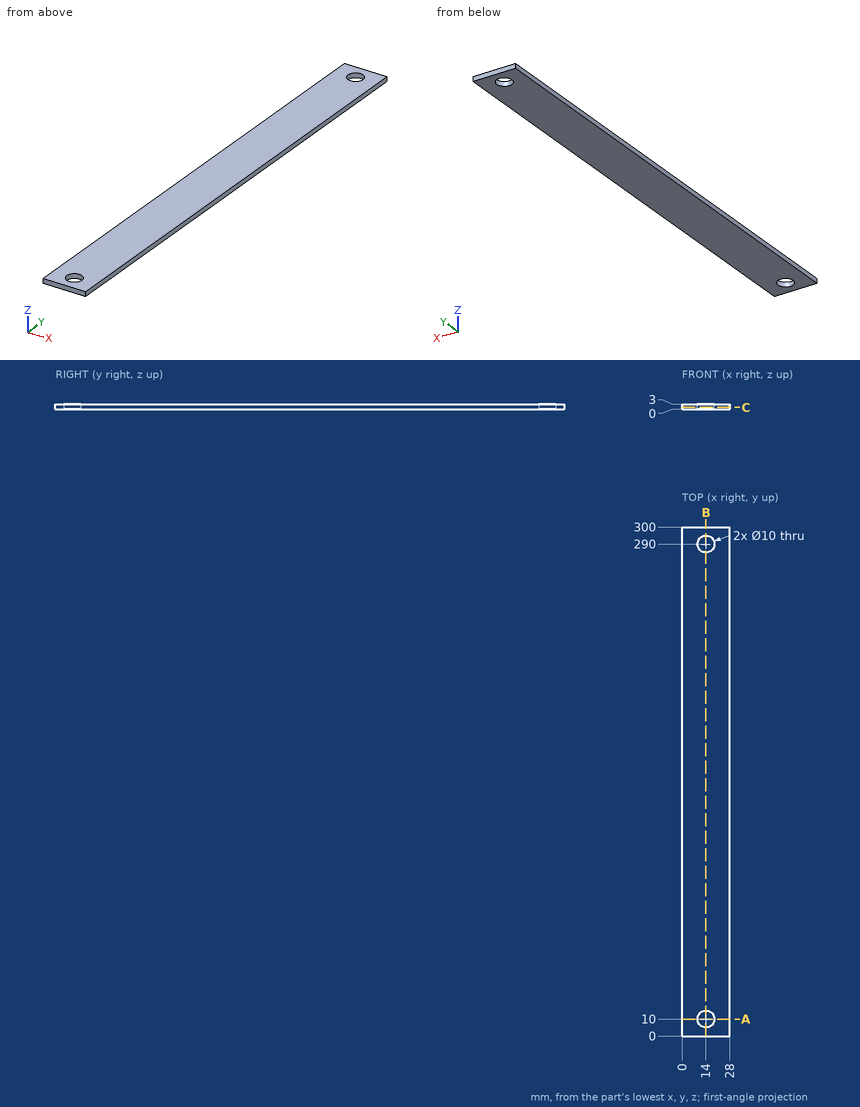
The figure shows three views and two pictorial views of one solid part (mm, origin at its lowest corner). Answer the questions. Give positions to 0.01 mm unless a question says otherwise; leave off trailing zeros. Write each loop counter-clockwise with the first axis right and the second up, starting at its lowest first coordinate (ties: lowest second). Pieces come first, ordered by that corner, then holes. Notation, with made-up numbers: (16.25, 55) -> (43.25, 55) arc R27 ccw to (43.25, 91) -> close; hole circle Ø2 at (41, -25.75). An arc over 180 degrees is marked (long way). Use one line per item in the form item = value.
1) Straight lines are drawn through the part: probe 1 along Y at (x, z) = (14, 1.95); probe 2 along X at (y, z) = (10, 0.95); probe 3 along Y at (x, z) = (13, 2.6). For each, find the intervals that lie inside material, in ascending order.
Result:
probe_1 = 0 to 5, 15 to 285, 295 to 300
probe_2 = 0 to 9, 19 to 28
probe_3 = 0 to 5.1, 14.9 to 285.1, 294.9 to 300
2) Section B-B on x = 14 is taken. Write down the section's boundary in (y, z).
Result:
outline = (0, 0) -> (5, 0) -> (5, 3) -> (0, 3) -> close; (15, 0) -> (285, 0) -> (285, 3) -> (15, 3) -> close; (295, 0) -> (300, 0) -> (300, 3) -> (295, 3) -> close
3) Section C-C on z = 1 is taken. Write down the section's boundary in (x, y), plus the area to 3 significant figures.
Result:
outline = (0, 0) -> (28, 0) -> (28, 300) -> (0, 300) -> close; hole circle Ø10 at (14, 10); hole circle Ø10 at (14, 290)
area = 8,240 mm²
4) Section A-A on y = 10 is taken. Write down the section's boundary in (x, z), plus the area to 3 significant figures.
Result:
outline = (0, 0) -> (9, 0) -> (9, 3) -> (0, 3) -> close; (19, 0) -> (28, 0) -> (28, 3) -> (19, 3) -> close
area = 54.0 mm²
